Work out the finished part from the listing and answer in its coordinate system (mm). Face numbers are marked on the shaded views. A direction names the side the tool comes from. Coordinates: 2 decimals unless noted, no trailing zeros. Order: outer loops, then holes, each group sorted by start corner. A loop starts at its lowest first (then second) coordinate and runs counter-clockwise, first axis right, second up. Notation, with made-up numbers: M 50.25,56.5 L 56.25,56.5 A29 ccw 56.25,79.5 Z; hole C 60.5,-5 d4. An arc over 180 degrees is marked long. Use a Markdown table: item, result.
from build123d import *

# Parameters (mm, degrees)
SKETCH1_W           = 203.2
SKETCH1_H           = 127
BOSS_EXTRUDE1_DEPTH = 6.35
SKETCH2_W           = 101.6
SKETCH2_H           = 101.6
SKETCH2_W_2         = 22.606
SKETCH2_H_2         = 3.302
CUT_EXTRUDE1_DEPTH  = 6.35
SKETCH3_W           = 203.2
SKETCH3_H           = 203.2
BOSS_EXTRUDE2_DEPTH = 6.35
SKETCH4_W           = 196.85
SKETCH4_H           = 127
BOSS_EXTRUDE3_DEPTH = 6.35
SKETCH5_W           = 190.5
SKETCH5_H           = 127
BOSS_EXTRUDE4_DEPTH = 6.35
SKETCH7_W           = 6.35
SKETCH7_H           = 190.5
BOSS_EXTRUDE5_DEPTH = 127
SKETCH8_R           = 5.3975
CUT_EXTRUDE2_DEPTH  = 6.35
SKETCH9_R           = 2.9972
CUT_EXTRUDE3_DEPTH  = 6.35


with BuildPart() as part:
    # Sketch1 → Boss-Extrude1 (new body)
    with BuildSketch(Plane.XY):
        with Locations((-101.6, 63.5)):
            Rectangle(SKETCH1_W, SKETCH1_H)
    extrude(amount=BOSS_EXTRUDE1_DEPTH)

    # Sketch2 → Cut-Extrude1 (cut)
    with BuildSketch(Plane.XY.offset(6.35)):
        with Locations((-64.77, 63.5)):
            Rectangle(SKETCH2_W, SKETCH2_H)
        with Locations((-159.385, 14.351)):
            Rectangle(SKETCH2_W_2, SKETCH2_H_2)
    extrude(amount=-CUT_EXTRUDE1_DEPTH, mode=Mode.SUBTRACT)

    # Sketch3 → Boss-Extrude2 (add)
    with BuildSketch(Plane.XZ):
        with Locations((-101.6, 101.6)):
            Rectangle(SKETCH3_W, SKETCH3_H)
    extrude(amount=BOSS_EXTRUDE2_DEPTH)

    # Sketch4 → Boss-Extrude3 (add)
    with BuildSketch(Plane.ZY.offset(203.2)):
        with Locations((104.775, 63.5)):
            Rectangle(SKETCH4_W, SKETCH4_H)
    boss_extrude3 = extrude(amount=-BOSS_EXTRUDE3_DEPTH)

    # Mirror1: Boss-Extrude3 across plane
    add(boss_extrude3.mirror(Plane(origin=(-101.6, 0, 0), x_dir=(0, 0, 1), z_dir=(1, 0, 0))))

    # Sketch5 → Boss-Extrude4 (add)
    with BuildSketch(Plane.XY.offset(203.2)):
        with Locations((-101.6, 63.5)):
            Rectangle(SKETCH5_W, SKETCH5_H)
    extrude(amount=-BOSS_EXTRUDE4_DEPTH)

    # Sketch7 → Boss-Extrude5 (add)
    with BuildSketch(Plane(origin=(0, 0, 0), x_dir=(1, 0, 0), z_dir=(0, 1, 0))):
        with Locations((-144.907, -101.6)):
            Rectangle(SKETCH7_W, SKETCH7_H)
    extrude(amount=BOSS_EXTRUDE5_DEPTH)

    # Sketch8 → Cut-Extrude2 (cut)
    with BuildSketch(Plane.XY.offset(203.2)):
        with Locations((-171.577, 5.7785)):
            Circle(SKETCH8_R)
    extrude(amount=-CUT_EXTRUDE2_DEPTH, mode=Mode.SUBTRACT)

    # Sketch9 → Cut-Extrude3 (cut)
    with BuildSketch(Plane(origin=(0, 0, 0), x_dir=(-1, 0, 0), z_dir=(0, 0, -1))):
        with Locations((168.021, 114.3)):
            Circle(SKETCH9_R)
        with Locations((180.721, 114.3)):
            Circle(SKETCH9_R)
    extrude(amount=-CUT_EXTRUDE3_DEPTH, mode=Mode.SUBTRACT)


solid = part.part
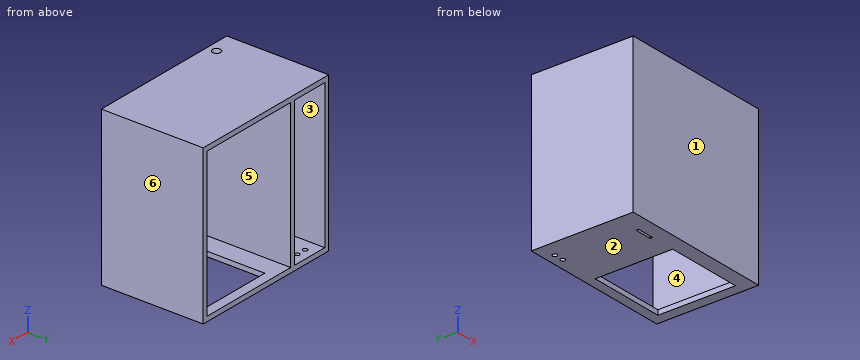
1. Find the intervals of material crossed by probe 1 along X at (y, z) = (67, 75); probe 2 along X at (y, z) = (114, 3); probe 3 along Z at (x, y) = (-120.5, 45.5), in increasing order.
Answers below:
| item | result |
|---|---|
| probe 1 | -203.2 to -196.85, -148.08 to -141.73, -6.35 to 0 |
| probe 2 | -203.2 to -183.7, -177.74 to -171, -165.04 to -115.57, -13.97 to 0 |
| probe 3 | 0 to 6.35, 196.85 to 203.2 |
2. Section A-A on x = -78.5 is taken. Determine the outline of the cut face in (y, z).
Answers below:
| item | result |
|---|---|
| outline | M -6.35,0 L 12.7,0 L 12.7,6.35 L 0,6.35 L 0,196.85 L 127,196.85 L 127,203.2 L -6.35,203.2 Z; M 114.3,0 L 127,0 L 127,6.35 L 114.3,6.35 Z |
3. Flat-ended cylindrical pins translate along their axes: P1, Ø5.5, axis at x = -168.021, y = 114.3, coming from the -Z side; P2, Ø10, axis at y = 46.5, z = 148, coming from the +X side. Find the tip coordinate at first contact, or state that the pin passes through.
Answers below:
| item | result |
|---|---|
| P1 | z = 196.85 |
| P2 | x = 0 |
4. For a pull along Z with two mould halves and no side action, classify the marked faces 1, 2, 3 and 4 as +Z half, -Z half, draft (parallel to the pull), parting line (faces both ways), or undercut.
Answers below:
| item | result |
|---|---|
| face 1 | draft |
| face 2 | -Z half |
| face 3 | undercut |
| face 4 | undercut |
5. Section C-C on z = 68 is taken. Determine the outline of the cut face in (x, y).
Answers below:
| item | result |
|---|---|
| outline | M -203.2,-6.35 L 0,-6.35 L 0,127 L -6.35,127 L -6.35,0 L -141.73,0 L -141.73,127 L -148.08,127 L -148.08,0 L -196.85,0 L -196.85,127 L -203.2,127 Z |
6. Section B-B on y = 19 is taken. Determine the outline of the cut face in (x, z).
Answers below:
| item | result |
|---|---|
| outline | M -203.2,0 L -115.57,0 L -115.57,6.35 L -141.73,6.35 L -141.73,196.85 L -6.35,196.85 L -6.35,6.35 L -13.97,6.35 L -13.97,0 L 0,0 L 0,203.2 L -203.2,203.2 Z; hole M -196.85,6.35 L -148.08,6.35 L -148.08,196.85 L -196.85,196.85 Z |
7. Section D-D on x = -127 is taken. Determine the outline of the cut face in (y, z).
Answers below:
| item | result |
|---|---|
| outline | M -6.35,0 L 127,0 L 127,6.35 L 0,6.35 L 0,196.85 L 127,196.85 L 127,203.2 L -6.35,203.2 Z |
8. For the marked faces 5 and 6, determine the directions among +Z, -Z, +X, -X, +Y, -Y from which every point of the face is accessible in a straight line to the end or side of a thin tool.
Answers below:
| item | result |
|---|---|
| face 5 | +Y |
| face 6 | +Z, -Z, +X, +Y, -Y |
